```python
from build123d import *

# Parameters (mm, degrees)
F0_R     = 2
F1_DEPTH = 0.5


with BuildPart() as f1:
    # F0 (on Top) → F1 (new body)
    with BuildSketch(Plane.XY):
        with BuildLine():
            ThreePointArc((31.75, 12.7), (29.890128, 17.190128), (25.4, 19.05))
            Line((25.4, 19.05), (-25.4, 19.05))
            ThreePointArc((-25.4, 19.05), (-29.890128, 17.190128), (-31.75, 12.7))
            Line((-31.75, 12.7), (-31.75, -12.7))
            ThreePointArc((-31.75, -12.7), (-29.890128, -17.190128), (-25.4, -19.05))
            Line((-25.4, -19.05), (25.4, -19.05))
            ThreePointArc((25.4, -19.05), (29.890128, -17.190128), (31.75, -12.7))
            Line((31.75, -12.7), (31.75, 12.7))
        make_face()
        with BuildLine():
            ThreePointArc((-22.5, -10.7), (-21.085786, -11.285786), (-20.5, -12.7))
            ThreePointArc((-20.5, -12.7), (-21.085786, -14.114214), (-22.5, -14.7))
            Line((-22.5, -14.7), (-27.5, -14.7))
            ThreePointArc((-27.5, -14.7), (-28.914214, -14.114214), (-29.5, -12.7))
            ThreePointArc((-29.5, -12.7), (-28.914214, -11.285786), (-27.5, -10.7))
            Line((-27.5, -10.7), (-22.5, -10.7))
        make_face(mode=Mode.SUBTRACT)
        with Locations((-12.7, -12.7)):
            Circle(F0_R, mode=Mode.SUBTRACT)
        with Locations((0, -12.7)):
            Circle(F0_R, mode=Mode.SUBTRACT)
        with Locations((12.7, -12.7)):
            Circle(F0_R, mode=Mode.SUBTRACT)
        with BuildLine():
            ThreePointArc((22.5, -14.7), (21.085786, -14.114214), (20.5, -12.7))
            ThreePointArc((20.5, -12.7), (21.085786, -11.285786), (22.5, -10.7))
            Line((22.5, -10.7), (27.5, -10.7))
            ThreePointArc((27.5, -10.7), (28.914214, -11.285786), (29.5, -12.7))
            ThreePointArc((29.5, -12.7), (28.914214, -14.114214), (27.5, -14.7))
            Line((27.5, -14.7), (22.5, -14.7))
        make_face(mode=Mode.SUBTRACT)
        with BuildLine():
            ThreePointArc((29.5, 0), (28.914214, -1.414214), (27.5, -2))
            Line((27.5, -2), (22.5, -2))
            ThreePointArc((22.5, -2), (21.085786, -1.414214), (20.5, 0))
            ThreePointArc((20.5, 0), (21.085786, 1.414214), (22.5, 2))
            Line((22.5, 2), (27.5, 2))
            ThreePointArc((27.5, 2), (28.914214, 1.414214), (29.5, 0))
        make_face(mode=Mode.SUBTRACT)
        with BuildLine():
            ThreePointArc((-27.5, -2), (-28.914214, -1.414214), (-29.5, 0))
            ThreePointArc((-29.5, 0), (-28.914214, 1.414214), (-27.5, 2))
            Line((-27.5, 2), (-22.5, 2))
            ThreePointArc((-22.5, 2), (-21.085786, 1.414214), (-20.5, 0))
            ThreePointArc((-20.5, 0), (-21.085786, -1.414214), (-22.5, -2))
            Line((-22.5, -2), (-27.5, -2))
        make_face(mode=Mode.SUBTRACT)
        with BuildLine():
            ThreePointArc((-22.5, 14.7), (-21.085786, 14.114214), (-20.5, 12.7))
            ThreePointArc((-20.5, 12.7), (-21.085786, 11.285786), (-22.5, 10.7))
            Line((-22.5, 10.7), (-27.5, 10.7))
            ThreePointArc((-27.5, 10.7), (-28.914214, 11.285786), (-29.5, 12.7))
            ThreePointArc((-29.5, 12.7), (-28.914214, 14.114214), (-27.5, 14.7))
            Line((-27.5, 14.7), (-22.5, 14.7))
        make_face(mode=Mode.SUBTRACT)
        with Locations((-12.7, 12.7)):
            Circle(F0_R, mode=Mode.SUBTRACT)
        Circle(F0_R, mode=Mode.SUBTRACT)
        with Locations((0, 12.7)):
            Circle(F0_R, mode=Mode.SUBTRACT)
        with Locations((12.7, 12.7)):
            Circle(F0_R, mode=Mode.SUBTRACT)
        with BuildLine():
            ThreePointArc((29.5, 12.7), (28.914214, 11.285786), (27.5, 10.7))
            Line((27.5, 10.7), (22.5, 10.7))
            ThreePointArc((22.5, 10.7), (21.085786, 11.285786), (20.5, 12.7))
            ThreePointArc((20.5, 12.7), (21.085786, 14.114214), (22.5, 14.7))
            Line((22.5, 14.7), (27.5, 14.7))
            ThreePointArc((27.5, 14.7), (28.914214, 14.114214), (29.5, 12.7))
        make_face(mode=Mode.SUBTRACT)
    extrude(amount=F1_DEPTH)


solid = f1.part
```
Source: CAD feature listing. Evaluate the final solid. Frame: model axes, mm. Round coordinates to 2 decimals unless told otherwise and drop trailing zeros. Loops run counter-clockwise (first coordinate to the right, second up) from the corner with the lowest first, then second, coordinate; pieces in that order, holes last. Notation, with made-up numbers: (-7, 19.25) - (38, 19.25) arc R15 cw to (38, 41.25) - close; hole circle Ø1 at (36.5, -1.5). An arc over 180 degrees is marked (long way). Use CSV: the item, a comma, the result in double quotes.
Q1. Mould query, pull axis Y, two halves, no side actions, for faces 1 (the cylindrical face through (29.84, -17.24, 0.25)), 2 (the cylindrical face through (-0.434, -1.952, 0.246)), 3 (the flat face through (0, 5, 0)), 4 (the cylindrical face through (-11.777, -14.474, 0.246)). Classes: pulls with the +Y half, pulls with the -Y half, needs draft (parallel to the pull), parting line crosses it, or undercut.
Reported:
face 1,"pulls with the -Y half"
face 2,"undercut"
face 3,"needs draft"
face 4,"undercut"
Q2. Pin query (flat end, axial travel): pin 1 Ø3 at (x, y) = (-12.7, 12.7) entering from +Z. Return the tip coordinate at first contact, or that it passes through.
Reported:
pin 1,"through"
Q3. Section query A-A, the plane x = 0. Output: boundary loops of the cut face in (y, z), then the cut area to 4 significant figures.
Reported:
outline,"(-19.05, 0) - (-14.7, 0) - (-14.7, 0.5) - (-19.05, 0.5) - close; (-10.7, 0) - (-2, 0) - (-2, 0.5) - (-10.7, 0.5) - close; (2, 0) - (10.7, 0) - (10.7, 0.5) - (2, 0.5) - close; (14.7, 0) - (19.05, 0) - (19.05, 0.5) - (14.7, 0.5) - close"
area,"13.05 mm^2"
Q4. Section query B-B, the plane x = 12.7. Output: boundary loops of the cut face in (y, z), then the cut area to 4 significant figures.
Reported:
outline,"(-19.05, 0) - (-14.7, 0) - (-14.7, 0.5) - (-19.05, 0.5) - close; (-10.7, 0) - (10.7, 0) - (10.7, 0.5) - (-10.7, 0.5) - close; (14.7, 0) - (19.05, 0) - (19.05, 0.5) - (14.7, 0.5) - close"
area,"15.05 mm^2"
Q5. Section query C-C, the plane z = 0.3. Give the number of separate pieces and of enclosed holes in the cut face, then the cut area to 3 significant figures.
Reported:
separate pieces,"1"
enclosed holes,"13"
area,"2,100 mm^2"
Q6. Ray query, line 1 along Y through (x, z) = (23.5, 0.45); line 2 along Y through (x, z) = (-12.7, 0.2); line 3 along Y through (x, z) = (1.5, 0.45). Return the intervals inside material, ascending.
Reported:
line 1,"-19.05 to -14.7, -10.7 to -2, 2 to 10.7, 14.7 to 19.05"
line 2,"-19.05 to -14.7, -10.7 to 10.7, 14.7 to 19.05"
line 3,"-19.05 to -14.02, -11.38 to -1.32, 1.32 to 11.38, 14.02 to 19.05"
